Could you check a few things on this model? Use its own coordinates, in mm. A direction names the side the tool comes from. Give positions to 0.01 mm unless a question says otherwise; leave off trailing zeros. Loops run counter-clockwise (first coordinate to the right, second up) from the corner with the lowest first, then second, coordinate; pieces in that order, holes last. Notation, with made-up numbers: (-10.75, 5) - (22.25, 5) arc R13 ccw to (22.25, 22) - close; hole circle Ø2 at (26, 34.25). An arc over 180 degrees is marked (long way). Write each question's results on one line, items separated by ' | '. Start each with the question number.
1) On a 3-axis mill with a long thin cutter (end or side, diameter ignored), from which of +Z, -Z, +X, -X, +Y, -Y can I reach the whole of each face in a straight line? I mean faces 5 (the face through (0, 157, 23.812)), 6 (the face through (11.3, 317.5, 2)). Say none if no direction works.
2) If we mould it in two halves opening along Z, with no side actions, what happens to faces 1 (the face through (-11.895, 140.948, -3.097)), 2 (the face through (0, 157, -25.4)), 3 (the face through (-11.112, 157, 0)), 4 (the face through (12.7, 157, 0))? For each: +Z half, -Z half, draft (parallel to the pull), parting line (faces both ways), or undercut.
3) I want a section at C-C, the plane y = 81.5. Write out the boundary of the cut face in (x, z), and give its area (3 significant figures).
4) If I drill on probe 1 along X at (y, z) = (298.5, 10.5); probe 2 along Z at (x, y) = (11.7, 127); probe 3 along Z at (x, y) = (9, 110.5), over which ranges is the centre line in solid material (lowest first)? Write a range as [from, to].
5) I want a section at A-A, the plane z = 18. Write out the boundary of the cut face in (x, y), and give its area (3 significant figures).
6) I want a section at D-D, the plane x = 8.5. Write out the boundary of the cut face in (y, z), and give its area (3 significant figures).
7) I want a section at B-B, the plane z = 0. Write out the boundary of the cut face in (x, y), and give its area (3 significant figures).
Autodesk Inventor part; units mm, degrees
ref_plane "YZ Plane" through (0, 0, 0) normal (1, 0, 0) x (0, 1, 0)
ref_plane "XZ Plane" through (0, 0, 0) normal (0, 1, 0) x (-1, 0, 0)
ref_plane "XY Plane" through (0, 0, 0) normal (0, 0, 1) x (1, 0, 0)
sketch "Sketch1" plane through (0, 0, 0) normal (0, 1, 0) x (-1, 0, 0)
  line L0 (-12.7, 25.4) -> (12.7, 25.4)
  line L1 (12.7, 25.4) -> (12.7, -25.4)
  line L2 (12.7, -25.4) -> (-12.7, -25.4)
  line L3 (-12.7, -25.4) -> (-12.7, 25.4)
  line L4 (-12.7, 25.4) -> (12.7, -25.4) construction
  line L5 (12.7, 25.4) -> (-12.7, -25.4) construction
  line L6 (11.1125, 23.8125) -> (-11.1125, 23.8125)
  line L7 (-11.1125, 23.8125) -> (-11.1125, -23.8125)
  line L8 (-11.1125, -23.8125) -> (11.1125, -23.8125)
  line L9 (11.1125, -23.8125) -> (11.1125, 23.8125)
  line L10 (11.1125, 23.8125) -> (-11.1125, -23.8125) construction
  line L11 (-11.1125, 23.8125) -> (11.1125, -23.8125) construction
  point P0 (0, 0)
  dimension "d0" = 25.4
  dimension "d1" = 50.8
  dimension "d2" = 22.225
  dimension "d3" = 47.625
extrude "Extrusion1" add sketch "Sketch1" along normal blind 317.5
sketch "Sketch2" plane through (-12.7, 0, -25.4) normal (-1, 0, 0) x (0, 0, 1)
  line L0 (50.8, 0) -> (50.8, 317.5)
  line L1 (0, 0) -> (50.8, 0)
  point P0 (25.4, 0)
  point P1 (25.4, 127)
  dimension "d13" = 25.4
  dimension "d14" = 127
hole "Hole1" at (-12.7, 127, 0) direction (1, 0, 0) diameter 28.575 end through all
properties part number "1x2 Frame" material "Aluminum 6061"
Answers:
1) face 5: +Y, -Y | face 6: +Z, -Z, +X, -X, +Y
2) face 1: undercut | face 2: -Z half | face 3: undercut | face 4: draft
3) outline: (-12.7, -25.4) - (12.7, -25.4) - (12.7, 25.4) - (-12.7, 25.4) - close; hole (-11.11, -23.81) - (11.11, -23.81) - (11.11, 23.81) - (-11.11, 23.81) - close | area: 232 mm2
4) probe 1: x = [-12.7, -11.11], [11.11, 12.7] | probe 2: z = [-25.4, -14.29], [14.29, 25.4] | probe 3: z = [-25.4, -23.81], [23.81, 25.4]
5) outline: (-12.7, 0) - (-11.11, 0) - (-11.11, 317.5) - (-12.7, 317.5) - close; (11.11, 0) - (12.7, 0) - (12.7, 317.5) - (11.11, 317.5) - close | area: 1,010 mm2
6) outline: (0, -25.4) - (317.5, -25.4) - (317.5, -23.81) - (0, -23.81) - close; (0, 23.81) - (317.5, 23.81) - (317.5, 25.4) - (0, 25.4) - close | area: 1,010 mm2
7) outline: (-12.7, 0) - (-11.11, 0) - (-11.11, 112.71) - (-12.7, 112.71) - close; (-12.7, 141.29) - (-11.11, 141.29) - (-11.11, 317.5) - (-12.7, 317.5) - close; (11.11, 0) - (12.7, 0) - (12.7, 112.71) - (11.11, 112.71) - close; (11.11, 141.29) - (12.7, 141.29) - (12.7, 317.5) - (11.11, 317.5) - close | area: 917 mm2
